Check sheet for the modelled part. Datum: model origin and axes. Units: mm. Face numbers are marked on the shaded views. A direction names the side the tool comes from. Round coordinates to 2 decimals unless told otherwise and drop trailing zeros. Order: outer loops, then holes, each group sorted by start corner. A loop starts at its lowest first (then second) coordinate and runs counter-clockwise, first axis right, second up. Notation, with made-up numbers: (87.5, 8) -> (136.5, 8) arc R29 cw to (136.5, 47) -> close; hole circle Ø9 at (51, 68.5). An arc over 180 degrees is marked (long way). Answer as CSV lines item,"result". Start each with the question number.
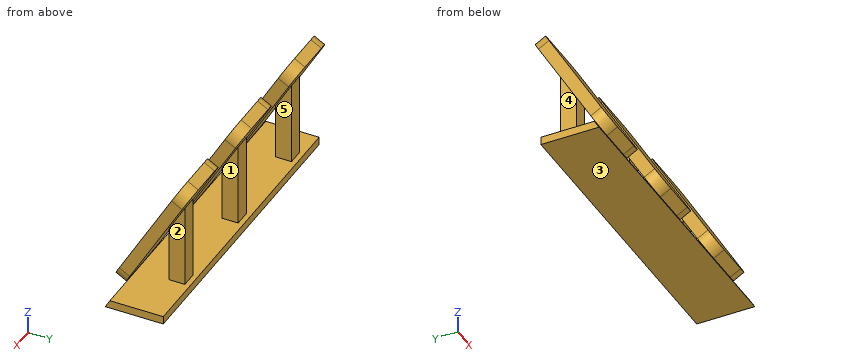
from build123d import *

# Parameters (mm, degrees)
SKETCH1_W           = 50
SKETCH1_H           = 30
BOSS_EXTRUDE1_DEPTH = 1
BOSS_EXTRUDE2_DEPTH = 50
SKETCH3_W           = 50
SKETCH3_H           = 20.262529014
SKETCH3_W_2         = 8
SKETCH3_H_2         = 17
CUT_EXTRUDE1_DEPTH  = 1.5
BOSS_EXTRUDE3_REACH = 18.249
SKETCH4_W           = 2
SKETCH4_H           = 2
CUT_EXTRUDE2_DEPTH  = 50
SKETCH6_W           = 12
SKETCH6_H           = 25.737309448
CUT_EXTRUDE3_DEPTH  = 1
SKETCH7_W           = 38
SKETCH7_H           = 17.625558307
CUT_EXTRUDE4_DEPTH  = 1
FILLET1_R           = 2
FILLET2_R           = 2


with BuildPart() as part:
    # Sketch1 → Boss-Extrude1 (new body)
    with BuildSketch(Plane.XY):
        Rectangle(SKETCH1_W, SKETCH1_H)
    extrude(amount=BOSS_EXTRUDE1_DEPTH)

    # Sketch2 → Boss-Extrude2 (add, through all)
    with BuildSketch(Plane(origin=(25, 0, 0), x_dir=(0, 0, -1), z_dir=(1, 0, 0))):
        Polygon((-1, -10.993105909), (-18.547864871, -0.861841403), (-17.797864871, 0.437196703), (-1, -9.261055102), align=None)
    extrude(amount=-BOSS_EXTRUDE2_DEPTH)

    # Sketch3 → Cut-Extrude1 (cut)
    with BuildSketch(Plane(origin=(0, -8.677842134, 5.010154492), x_dir=(1, 0, 0), z_dir=(0, -0.866025404, 0.5))):
        with Locations((0, 5.500736956)):
            Rectangle(SKETCH3_W, SKETCH3_H)
        with Locations((19, 5.632001463)):
            Rectangle(SKETCH3_W_2, SKETCH3_H_2, mode=Mode.SUBTRACT)
        with Locations((6, 5.632001463)):
            Rectangle(SKETCH3_W_2, SKETCH3_H_2, mode=Mode.SUBTRACT)
        with Locations((-7, 5.632001463)):
            Rectangle(SKETCH3_W_2, SKETCH3_H_2, mode=Mode.SUBTRACT)
    extrude(amount=-CUT_EXTRUDE1_DEPTH, mode=Mode.SUBTRACT)

    # Boss-Extrude3: up to this face of the body (flat: up to its plane)
    boss_extrude3_end = Plane(part.part.faces().sort_by_distance((19, -5.861841403, 9.887610833))[0])
    # Sketch4 → Boss-Extrude3 (add, up to the picked face)
    with BuildSketch(Plane.XY.offset(1), mode=Mode.PRIVATE) as boss_extrude3_sk1:
        with Locations((17.490902079, -4.261055102)):
            Rectangle(SKETCH4_W, SKETCH4_H)
    boss_extrude3_tool1 = split(extrude(boss_extrude3_sk1.sketch, amount=BOSS_EXTRUDE3_REACH, mode=Mode.PRIVATE), bisect_by=boss_extrude3_end, keep=Keep.BOTH, mode=Mode.PRIVATE)
    add(boss_extrude3_tool1.solids().sort_by_distance((17.490902, -4.261055, 1))[0])
    # Sketch4 → Boss-Extrude3 (add, up to the picked face)
    with BuildSketch(Plane.XY.offset(1), mode=Mode.PRIVATE) as boss_extrude3_sk2:
        with Locations((4.490902079, -4.261055102)):
            Rectangle(SKETCH4_W, SKETCH4_H)
    boss_extrude3_tool2 = split(extrude(boss_extrude3_sk2.sketch, amount=BOSS_EXTRUDE3_REACH, mode=Mode.PRIVATE), bisect_by=boss_extrude3_end, keep=Keep.BOTH, mode=Mode.PRIVATE)
    add(boss_extrude3_tool2.solids().sort_by_distance((4.490902, -4.261055, 1))[0])
    # Sketch4 → Boss-Extrude3 (add, up to the picked face)
    with BuildSketch(Plane.XY.offset(1), mode=Mode.PRIVATE) as boss_extrude3_sk3:
        with Locations((-8.509097921, -4.261055102)):
            Rectangle(SKETCH4_W, SKETCH4_H)
    boss_extrude3_tool3 = split(extrude(boss_extrude3_sk3.sketch, amount=BOSS_EXTRUDE3_REACH, mode=Mode.PRIVATE), bisect_by=boss_extrude3_end, keep=Keep.BOTH, mode=Mode.PRIVATE)
    add(boss_extrude3_tool3.solids().sort_by_distance((-8.509098, -4.261055, 1))[0])

    # Sketch5 → Cut-Extrude2 (cut)
    with BuildSketch(Plane.ZY.offset(25)):
        Polygon((0.250581886, -9.69507566), (0, -9.840198507), (0, -15), (1, -15), (1, -10.993105909), align=None)
    extrude(amount=-CUT_EXTRUDE2_DEPTH, mode=Mode.SUBTRACT)

    # Sketch6 → Cut-Extrude3 (cut)
    with BuildSketch(Plane.XY.offset(1)):
        with Locations((-19, 2.131345276)):
            Rectangle(SKETCH6_W, SKETCH6_H)
    extrude(amount=-CUT_EXTRUDE3_DEPTH, mode=Mode.SUBTRACT)

    # Sketch7 → Cut-Extrude4 (cut)
    with BuildSketch(Plane.XY.offset(1)):
        with Locations((6, 6.187220847)):
            Rectangle(SKETCH7_W, SKETCH7_H)
    extrude(amount=-CUT_EXTRUDE4_DEPTH, mode=Mode.SUBTRACT)

    # Fillet1
    fillet1_edges = [part.edges().sort_by_distance(p)[0] for p in [
        (-3, -9.46232235, 2.151394901),
        (-3, -0.96232235, 16.873826765),
        (-11, -0.96232235, 16.873826765),
        (-11, -9.46232235, 2.151394901),
    ]]
    fillet(fillet1_edges, radius=FILLET1_R)

    # Fillet2
    fillet2_edges = [part.edges().sort_by_distance(p)[0] for p in [
        (23, -9.46232235, 2.151394901),
        (23, -0.96232235, 16.873826765),
        (15, -0.96232235, 16.873826765),
        (15, -9.46232235, 2.151394901),
        (10, -9.46232235, 2.151394901),
        (10, -0.96232235, 16.873826765),
        (2, -0.96232235, 16.873826765),
        (2, -9.46232235, 2.151394901),
    ]]
    fillet(fillet2_edges, radius=FILLET2_R)


solid = part.part
1) Section check D-D on y = -4.75. Record the cut outline in (x, z).
2) Material ranges on line 1 along X through (y, z) = (-4, 8); line 2 along X through (y, z) = (-8, 5.25); line 3 along Z through (x, y) = (10.5, -7), recorded low to high.
3) Section check C-C on z = 5. Record the cut outline in (x, y), then the cut area to 3 significant figures.
4) Mould release check, pull along X, two halves, no side actions. Record for the marked faces 1, 2 and 3: released by +X, released by -X, zero draft, split by the parting line, or undercut.
5) Access from +Z, -Z, +X, -X, +Y, -Y to the whole of each face (thin tool, end or side, straight path). Record for the marked faces 4 and 5.
6) Section check A-A on z = 8.5. Record the cut outline in (x, y).
7) Depth check by flat-ended pin: pin 1 Ø0.5 at (x, z) = (-1, 0.5) entering from +Y; pin 2 Ø4 at (y, z) = (-4, 9) entering from -X; pin 3 Ø10 at (x, z) = (2.5, 7) entering from +Y; pin 4 Ø2 at (y, z) = (-6.5, 13) entering from +X. Enter the tip coordinate at first touch or a pass-through.
Solutions:
1,outline,"(-13, 0) -> (25, 0) -> (25, 1) -> (18.49, 1) -> (18.49, 8.81) -> (23, 8.81) -> (23, 11.81) -> (15, 11.81) -> (15, 8.81) -> (16.49, 8.81) -> (16.49, 1) -> (5.49, 1) -> (5.49, 8.81) -> (10, 8.81) -> (10, 11.81) -> (2, 11.81) -> (2, 8.81) -> (3.49, 8.81) -> (3.49, 1) -> (-7.51, 1) -> (-7.51, 8.81) -> (-3, 8.81) -> (-3, 11.81) -> (-11, 11.81) -> (-11, 8.81) -> (-9.51, 8.81) -> (-9.51, 1) -> (-13, 1) -> close"
2,line 1,"x = -9.51 to -7.51, 3.49 to 5.49, 16.49 to 18.49"
2,line 2,"x = -11 to -3, 2 to 10, 15 to 23"
2,line 3,"z = 0 to 1"
3,outline,"(-11, -8.68) -> (-3, -8.68) -> (-3, -6.95) -> (-11, -6.95) -> close; (-9.51, -5.26) -> (-7.51, -5.26) -> (-7.51, -3.26) -> (-9.51, -3.26) -> close; (2, -8.68) -> (10, -8.68) -> (10, -6.95) -> (2, -6.95) -> close; (3.49, -5.26) -> (5.49, -5.26) -> (5.49, -3.26) -> (3.49, -3.26) -> close; (15, -8.68) -> (23, -8.68) -> (23, -6.95) -> (15, -6.95) -> close; (16.49, -5.26) -> (18.49, -5.26) -> (18.49, -3.26) -> (16.49, -3.26) -> close"
3,area,"53.6 mm^2"
4,face 1,"undercut"
4,face 2,"released by +X"
4,face 3,"zero draft"
5,face 4,"-X, +Y"
5,face 5,"+Y"
6,outline,"(-11, -6.66) -> (-3, -6.66) -> (-3, -4.93) -> (-7.51, -4.93) -> (-7.51, -3.26) -> (-9.51, -3.26) -> (-9.51, -4.93) -> (-11, -4.93) -> close; (2, -6.66) -> (10, -6.66) -> (10, -4.93) -> (5.49, -4.93) -> (5.49, -3.26) -> (3.49, -3.26) -> (3.49, -4.93) -> (2, -4.93) -> close; (15, -6.66) -> (23, -6.66) -> (23, -4.93) -> (18.49, -4.93) -> (18.49, -3.26) -> (16.49, -3.26) -> (16.49, -4.93) -> (15, -4.93) -> close"
7,pin 1,"stops at y = -2.63"
7,pin 2,"stops at x = -11"
7,pin 3,"stops at y = -2.91"
7,pin 4,"passes through"
